from build123d import *

# Parameters (mm, degrees)
BOSS_EXTRUDE1_DEPTH = 11.5
SHELL1_T            = -3
SKETCH3_R           = 1.3
CUT_EXTRUDE1_DEPTH  = 94
SKETCH4_R           = 1.3
CUT_EXTRUDE2_DEPTH  = 94
FILLET1_R           = 2
CUT_EXTRUDE3_DEPTH  = 79
CUT_EXTRUDE4_DEPTH  = 79
FILLET2_R           = 2
SKETCH7_R           = 1.6
CUT_EXTRUDE5_DEPTH  = 10
SKETCH8_R           = 1
CUT_EXTRUDE7_DEPTH  = 79
CUT_EXTRUDE8_DEPTH  = 1.5
CUT_EXTRUDE9_DEPTH  = 1.5
FILLET3_R           = 1
CUT_EXTRUDE10_DEPTH = 10
FILLET4_R           = 1
SKETCH14_R          = 1.6
CUT_EXTRUDE11_DEPTH = 10


with BuildPart() as part:
    # Sketch1 → Boss-Extrude1 (new body)
    with BuildSketch(Plane(origin=(0, 0, 0), x_dir=(1, 0, 0), z_dir=(0, 1, 0))):
        Polygon((-11.213203436, 40), (18.786796564, 40), (40, 18.786796564), (40, -11.213203436), (18.786796564, -32.426406871), (-11.213203436, -32.426406871), (-32.426406871, -11.213203436), (-32.426406871, 18.786796564), align=None)
    extrude(amount=BOSS_EXTRUDE1_DEPTH)

    # Shell1
    shell1_openings = [part.faces().sort_by_distance(p)[0] for p in [
        (3.786796564, 11.5, -3.786796564),
    ]]
    offset(amount=SHELL1_T, openings=shell1_openings, kind=Kind.INTERSECTION)

    # Sketch3 → Cut-Extrude1 (cut)
    with BuildSketch(Plane(origin=(-21.819805153, 0, 21.819805153), x_dir=(0.7071067811865558, 0, 0.7071067811865392), z_dir=(-0.7071067811865392, 0, 0.7071067811865558))):
        with Locations((-9, 7.25)):
            Circle(SKETCH3_R)
        with Locations((9, 7.25)):
            Circle(SKETCH3_R)
    extrude(amount=-CUT_EXTRUDE1_DEPTH, mode=Mode.SUBTRACT)

    # Sketch4 → Cut-Extrude2 (cut)
    with BuildSketch(Plane(origin=(-25.606601718, 0, -25.606601718), x_dir=(-0.7071067811865556, 0, 0.7071067811865396), z_dir=(-0.7071067811865396, 0, -0.7071067811865556))):
        with Locations((-14.355339059, 7.25)):
            Circle(SKETCH4_R)
        with Locations((3.644660941, 7.25)):
            Circle(SKETCH4_R)
    extrude(amount=-CUT_EXTRUDE2_DEPTH, mode=Mode.SUBTRACT)

    # Fillet1
    fillet1_edges = [part.edges().sort_by_distance(p)[0] for p in [
        (40, 5.75, -18.786796564),
        (40, 5.75, 11.213203436),
        (18.786796564, 5.75, 32.426406871),
        (-11.213203436, 5.75, 32.426406871),
        (-32.426406871, 5.75, 11.213203436),
        (-32.426406871, 5.75, -18.786796564),
        (-11.213203436, 5.75, -40),
        (18.786796564, 5.75, -40),
    ]]
    fillet(fillet1_edges, radius=FILLET1_R)

    # Sketch5 → Cut-Extrude3 (cut)
    with BuildSketch(Plane.XY.offset(32.426406871)):
        Polygon((3.786796564, 7), (13.286796564, 7), (13.286796564, 11.5), (-5.713203436, 11.5), (-5.713203436, 7), align=None)
    extrude(amount=-CUT_EXTRUDE3_DEPTH, mode=Mode.SUBTRACT)

    # Sketch6 → Cut-Extrude4 (cut)
    with BuildSketch(Plane.ZY.offset(32.426406871)):
        Polygon((-3.786796564, 7), (5.713203436, 7), (5.713203436, 11.5), (-13.286796564, 11.5), (-13.286796564, 7), align=None)
    extrude(amount=-CUT_EXTRUDE4_DEPTH, mode=Mode.SUBTRACT)

    # Fillet2
    fillet2_edges = [part.edges().sort_by_distance(p)[0] for p in [
        (-5.713203436, 7, -38.5),
        (-5.713203436, 11.5, -38.5),
        (13.286796564, 11.5, -38.5),
        (13.286796564, 7, -38.5),
        (-5.713203436, 7, 30.926406871),
        (-5.713203436, 11.5, 30.926406871),
        (13.286796564, 11.5, 30.926406871),
        (13.286796564, 7, 30.926406871),
        (38.5, 7, -13.286796564),
        (-30.926406871, 7, -13.286796564),
        (38.5, 11.5, -13.286796564),
        (-30.926406871, 11.5, -13.286796564),
        (38.5, 11.5, 5.713203436),
        (-30.926406871, 11.5, 5.713203436),
        (38.5, 7, 5.713203436),
        (-30.926406871, 7, 5.713203436),
    ]]
    fillet(fillet2_edges, radius=FILLET2_R)

    # Sketch7 → Cut-Extrude5 (cut)
    with BuildSketch(Plane(origin=(0, 0, 0), x_dir=(-1, 0, 0), z_dir=(0, -1, 0))):
        with Locations(Location((6.213203436, -6.213203436, 0), (0, 0, 90))):
            Circle(SKETCH7_R)
        with Locations(Location((-13.786796564, -6.213203436, 0), (0, 0, 90))):
            Circle(SKETCH7_R)
        with Locations(Location((-13.786796564, 13.786796564, 0), (0, 0, 90))):
            Circle(SKETCH7_R)
        with Locations(Location((6.213203436, 13.786796564, 0), (0, 0, 90))):
            Circle(SKETCH7_R)
    extrude(amount=-CUT_EXTRUDE5_DEPTH, mode=Mode.SUBTRACT)

    # Sketch8 → Cut-Extrude7 (cut)
    with BuildSketch(Plane(origin=(40, 0, 0), x_dir=(0, 0, -1), z_dir=(1, 0, 0))):
        with Locations((-8.213203436, 10)):
            Circle(SKETCH8_R)
        with Locations((-8.213203436, 3)):
            Circle(SKETCH8_R)
        with Locations((15.786796564, 3)):
            Circle(SKETCH8_R)
        with Locations(Location((15.786796564, 10, 0), (0, 0, 180))):
            Circle(SKETCH8_R)
    extrude(amount=-CUT_EXTRUDE7_DEPTH, mode=Mode.SUBTRACT)

    # Sketch10 → Cut-Extrude8 (cut)
    with BuildSketch(Plane(origin=(0, 3, 0), x_dir=(1, 0, 0), z_dir=(0, 1, 0))):
        Polygon((17.544155877, 37), (37, 17.544155877), (37, -9.970562748), (17.544155877, -29.426406871), (-9.970562748, -29.426406871), (-29.426406871, -9.970562748), (-29.426406871, 17.544155877), (-9.970562748, 37), align=None)
    extrude(amount=-CUT_EXTRUDE8_DEPTH, mode=Mode.SUBTRACT)

    # Sketch12 → Cut-Extrude9 (cut)
    with BuildSketch(Plane(origin=(0, 1.5, 0), x_dir=(1, 0, 0), z_dir=(0, 1, 0))):
        Polygon((-26.426406871, 20.544155877), (-29.426406871, 17.544155877), (-29.426406871, 12.286796564), (-26.426406871, 12.286796564), align=None)
        Polygon((-26.426406871, -4.713203436), (-29.426406871, -4.713203436), (-29.426406871, -9.970562748), (-26.426406871, -12.970562748), align=None)
        Polygon((34, 12.286796564), (37, 12.286796564), (37, 17.544155877), (34, 20.544155877), align=None)
        Polygon((37, -9.970562748), (37, -4.713203436), (34, -4.713203436), (34, -12.970562748), align=None)
    extrude(amount=-CUT_EXTRUDE9_DEPTH, mode=Mode.SUBTRACT)

    # Fillet3
    fillet3_edges = [part.edges().sort_by_distance(p)[0] for p in [
        (-26.426406871, 0.75, 4.713203436),
        (-26.426406871, 0.75, 12.970562748),
        (-29.426406871, 0.75, 4.713203436),
        (34, 0.75, -12.286796564),
        (34, 0.75, -20.544155877),
        (37, 0.75, -12.286796564),
        (37, 0.75, 4.713203436),
        (34, 0.75, 12.970562748),
        (34, 0.75, 4.713203436),
        (-29.426406871, 0.75, -12.286796564),
        (-26.426406871, 0.75, -20.544155877),
        (-26.426406871, 0.75, -12.286796564),
    ]]
    fillet(fillet3_edges, radius=FILLET3_R)

    # Sketch13 → Cut-Extrude10 (cut)
    with BuildSketch(Plane(origin=(0, 1.5, 0), x_dir=(1, 0, 0), z_dir=(0, 1, 0))):
        Polygon((3.786796564, 19.838268012), (-4.213203436, 19.838268012), (-4.213203436, 32.838268012), (2.581997553, 32.838268012), (11.786796564, 32.838268012), (11.786796564, 19.838268012), align=None)
        Polygon((19.838268012, 3.786796564), (19.838268012, -4.213203436), (32.838268012, -4.213203436), (32.838268012, 4.991595576), (32.838268012, 11.786796564), (19.838268012, 11.786796564), align=None)
        Polygon((3.786796564, -12.264674884), (-4.213203436, -12.264674884), (-4.213203436, -25.264674884), (4.991595576, -25.264674884), (11.786796564, -25.264674884), (11.786796564, -12.264674884), align=None)
        Polygon((-12.264674884, 3.786796564), (-12.264674884, 11.786796564), (-25.264674884, 11.786796564), (-25.264674884, 2.581997553), (-25.264674884, -4.213203436), (-12.264674884, -4.213203436), align=None)
    extrude(amount=-CUT_EXTRUDE10_DEPTH, mode=Mode.SUBTRACT)

    # Fillet4
    fillet4_edges = [part.edges().sort_by_distance(p)[0] for p in [
        (11.786796564, 0.75, -19.838268012),
        (-4.213203436, 0.75, -19.838268012),
        (-4.213203436, 0.75, -32.838268012),
        (11.786796564, 0.75, -32.838268012),
        (19.838268012, 0.75, -11.786796564),
        (32.838268012, 0.75, -11.786796564),
        (32.838268012, 0.75, 4.213203436),
        (19.838268012, 0.75, 4.213203436),
        (11.786796564, 0.75, 12.264674884),
        (11.786796564, 0.75, 25.264674884),
        (-4.213203436, 0.75, 25.264674884),
        (-4.213203436, 0.75, 12.264674884),
        (-12.264674884, 0.75, 4.213203436),
        (-25.264674884, 0.75, 4.213203436),
        (-25.264674884, 0.75, -11.786796564),
        (-12.264674884, 0.75, -11.786796564),
    ]]
    fillet(fillet4_edges, radius=FILLET4_R)

    # Sketch14 → Cut-Extrude11 (cut)
    with BuildSketch(Plane(origin=(0, 1.5, 0), x_dir=(1, 0, 0), z_dir=(0, 1, 0))):
        with Locations(Location((-14.597979746, 22.171572875, 0), (0, 0, 270))):
            Circle(SKETCH14_R)
        with Locations(Location((22.171572875, 22.171572875, 0), (0, 0, 270))):
            Circle(SKETCH14_R)
        with Locations(Location((-14.597979746, -14.597979746, 0), (0, 0, 270))):
            Circle(SKETCH14_R)
        with Locations(Location((22.171572875, -14.597979746, 0), (0, 0, 270))):
            Circle(SKETCH14_R)
    extrude(amount=-CUT_EXTRUDE11_DEPTH, mode=Mode.SUBTRACT)


solid = part.part
Source: CAD feature listing. Evaluate the final solid. Frame: model axes, mm. A direction names the side the tool comes from. Coordinates: 2 decimals unless noted, no trailing zeros. Order: outer loops, then holes, each group sorted by start corner. A loop starts at its lowest first (then second) coordinate and runs counter-clockwise, first axis right, second up. Notation, with made-up numbers: M 9,-36 L 52,-36 A11 cw 52,-20 Z; hole C -11,75 d1. An arc over 180 degrees is marked long. Write each question's results on one line, items separated by ' | '. Start each with the question number.
1. Reachability of faces 1 (the face through (4, 7, 31)), 2 (the face through (27.136, 5.67, -27.408)), 3 (the face through (-30.905, 7.601, -12.716)) from +Z, -Z, +X, -X, +Y, -Y: full face, straight path, thin tool, end or side. Return the list, or none.
2. Section C-C, the plane x = -18. Return the cut outline in (y, z), then the cut area to 3 significant figures.
3. Section B-B, the plane z = 19. Return the cut outline in (x, y), then the cut area to 3 significant figures.
4. Draft query along X for faces 4 (the face through (-29.426, 5, -4)), 5 (the face through (-32.426, 4, -4)), 6 (the face through (-30.91, 10.3, 7.26)). Return one class per face: +X half, -X half, draft (parallel to the pull), parting line (faces both ways), or undercut.
5. Pin query (flat end, axial travel): pin 1 (0.8 mm diameter, centred on x = 27, y = 1, fed in from +Z); pin 2 (8 mm diameter, centred on x = 25, z = 23.5, fed in from -Y); pin 3 (3 mm diameter, centred on x = -14.5, y = 8, fed in from +Z); pin 4 (1.5 mm diameter, centred on y = 3.5, z = -19.5, fed in from -X). Return the tip coordinate at first contact, or that it passes through.
6. Section A-A, the plane x = 1. Return the cut outline in (y, z), then the cut area to 3 significant figures.
7. Material intervals for L1, parallel to X at y = 0.75, z = 9; L2, parallel to Z at x = -2.5, y = 6.5; L3, parallel to X at y = 6.75, z = 7, sorted ascending.
Solution:
1) face 1: +Z, -Z, +Y | face 2: +Y | face 3: +X, -X, +Y
2) outline: M 0,-33.21 L 11.5,-33.21 L 11.5,-28.97 L 1.5,-28.97 L 1.5,-11.79 L 0,-11.79 Z; M 0,4.21 L 1.5,4.21 L 1.5,21.4 L 11.5,21.4 L 11.5,25.64 L 0,25.64 Z | area: 149 mm²
3) outline: M -24.64,0 L -4.21,0 L -4.21,1.5 L -20.4,1.5 L -20.4,11.5 L -24.64,11.5 Z; M 11.79,0 L 32.21,0 L 32.21,11.5 L 27.97,11.5 L 27.97,1.5 L 11.79,1.5 Z | area: 146 mm²
4) face 4: undercut | face 5: -X half | face 6: draft
5) pin 1: z = 24.61 | pin 2: y = 0 | pin 3: z = 30.64 | pin 4: x = -32.26
6) outline: M 0,-40 L 7,-40 L 7,-37 L 1.5,-37 L 1.5,-32.84 L 0,-32.84 Z; M 0,-19.84 L 1.5,-19.84 L 1.5,12.26 L 0,12.26 Z; M 0,25.26 L 1.5,25.26 L 1.5,29.43 L 7,29.43 L 7,32.43 L 0,32.43 Z | area: 103 mm²
7) L1: -32.43 to -29.43, -26.43 to 34, 37 to 40 | L2: -40 to -37, 29.43 to 32.43 | L3: -32.43 to -29.43, 37 to 40
